Check sheet for the modelled part. Datum: model origin and axes. Units: mm. A direction names the side the tool comes from. Coordinates: 2 decimals unless noted, no trailing zeros. Loops run counter-clockwise (first coordinate to the right, second up) from the corner with the lowest first, then second, coordinate; pieces in that order, holes last. Notation, with made-up numbers: (62.5, 13) - (99.5, 13) arc R22 cw to (99.5, 42) - close; hole circle Ø11 at (50.25, 38.25). An arc over 180 degrees is marked (long way). Use a Markdown table: item, result. Add a question column.
1) Sectioned sample at B-B, the plane y = -153. Enter the section's corners in (x, z).
2) Sectioned sample at A-A, the plane z = 212.5. Enter the section's corners in (x, y).
3) Tool access check on faces 1 (the flat face through (-390, -148, 142)), 2 (the flat face through (-385, -148, 144)). Record the directions out of +Z, -Z, +X, -X, +Y, -Y that give a thin tool (end or side, any length) a straight path to the whole face; none if there is none.
4) Draft check along Z on faces 3 (the flat face through (5, 32.73, 203)), 4 (the flat face through (5, -148, 0)), 5 (the flat face through (390, -148, 146)). Enter one of: pulls with the +Z half, pulls with the -Z half, needs draft (parallel to the pull), parting line crosses it, or undercut.
5) Thickness scan on line 1 (Z direction, x = 12.5, y = -230); line 2 (Y direction, x = -308, z = 250.5); line 3 (X direction, y = -125.5, z = 29). Record the ranges inside material, lowest first.
6) Go/stop test with flat-tipped pins: P1, Ø3.5, axis at x = -2, y = 34, coming from the -Z side; P2, Ø1.5, axis at x = 182, y = -252.5, coming from the +Z side; P3, Ø5, axis at y = -7.5, z = 299, coming from the +X side. Record where each tip stops, or that it passes through.
from build123d import *

# Parameters (mm, degrees)
EXTRUDE_START            = -329.393398282
EXTRUDE_1_DEPTH          = 367.123106012
CUT_EXTRUDE_2_REACH      = 654.668
CUT_EXTRUDE_2_END_RADIUS = 675
SKETCH_4_W               = 770
SKETCH_4_H               = 357.123106012
SKETCH_5_RX              = 84.852813742
SKETCH_5_RY              = 60
CUT_EXTRUDE_3_DEPTH      = 10


# Read off the part's stored shape, not the designer's step: 凸台-拉伸1
with BuildPart() as part:
    # 凸台-拉伸1 outline → 凸台-拉伸1 (new body)
    with BuildSketch(Plane(origin=(0, 0, 0), x_dir=(1, 0, 0), z_dir=(0, 1, 0)).offset(EXTRUDE_START)):
        with BuildLine():
            Line((390, -288.70946964), (390, 0))
            Line((390, 0), (-390, 0))
            Line((-390, 0), (-390, -288.70946964))
            ThreePointArc((-390, -288.70946964), (0, -411.663690552), (390, -288.70946964))
        make_face()
    extrude(amount=EXTRUDE_1_DEPTH)

    # 切除-拉伸2: up to this cylinder (the profile starts inside it)
    cut_extrude_2_end = Plane(origin=(0, -145.831845, -268.336309448), z_dir=(0, 1, 0)) * Cylinder(CUT_EXTRUDE_2_END_RADIUS, 2660.336, mode=Mode.PRIVATE)
    # 草图4 → 切除-拉伸2 (cut, up to the surface)
    with BuildSketch(Plane(origin=(0, 0, 5), x_dir=(-1, 0, 0), z_dir=(0, 0, -1)), mode=Mode.PRIVATE) as cut_extrude_2_sk1:
        with Locations((0, -145.831845276)):
            Rectangle(SKETCH_4_W, SKETCH_4_H)
    cut_extrude_2_tool1 = extrude(cut_extrude_2_sk1.sketch, amount=-CUT_EXTRUDE_2_REACH, mode=Mode.PRIVATE) & cut_extrude_2_end
    add(cut_extrude_2_tool1.solids().sort_by_distance((0, -145.831845, 5))[0], mode=Mode.SUBTRACT)

    # 草图5 → 切除-拉伸3 (cut)
    with BuildSketch(Plane(origin=(0, 0, 0), x_dir=(-1, 0, 0), z_dir=(0, 0, -1))):
        with Locations(Location((0, -47.72970773), (0, 0, 90))):
            Ellipse(SKETCH_5_RX, SKETCH_5_RY)
    extrude(amount=-CUT_EXTRUDE_3_DEPTH, mode=Mode.SUBTRACT)


solid = part.part
Solved:
| question | item | result |
|---|---|---|
| 1 | outline | (-390, 0) - (390, 0) - (390, 288.71) arc R680 ccw to (-390, 288.71) - close; hole (-385, 5) - (385, 5) - (385, 286.1) arc R675 ccw to (-385, 286.1) - close |
| 2 | outline | (-390, -329.39) - (390, -329.39) - (390, 37.73) - (-390, 37.73) - close; hole (-385, -324.39) - (385, -324.39) - (385, 32.73) - (-385, 32.73) - close |
| 3 | face 1 | +Z, -Z, -X, +Y, -Y |
| 3 | face 2 | none |
| 4 | face 3 | undercut |
| 4 | face 4 | pulls with the -Z half |
| 4 | face 5 | needs draft |
| 5 | line 1 | z = 0 to 5, 406.55 to 411.55 |
| 5 | line 2 | y = -329.39 to -324.39, 32.73 to 37.73 |
| 5 | line 3 | x = -390 to -385, 385 to 390 |
| 6 | P1 | stops at z = 10 |
| 6 | P2 | stops at z = 387.06 |
| 6 | P3 | stops at x = 378.63 |
